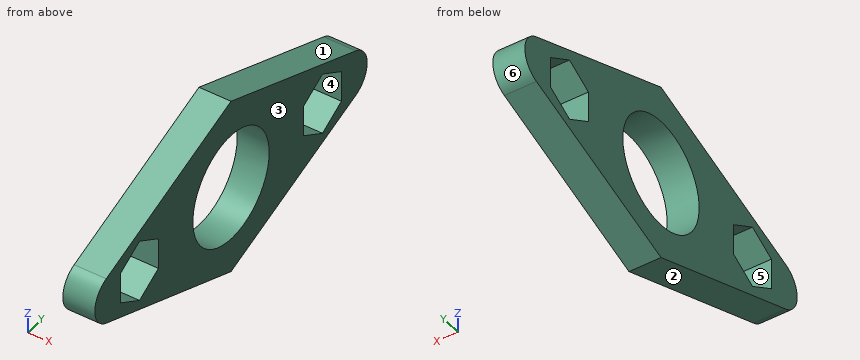
```python
from build123d import *

# Parameters (mm, degrees)
F0_R     = 10.9
F1_DEPTH = 6.35
F2_R     = 5


with BuildPart() as f1:
    # F0 (on Right) → F1 (new body)
    with BuildSketch(Plane.YZ):
        Polygon((48.273511, 0), (0, 18.102249), (-48.273511, 0), (0, -17.76745), align=None)
        Polygon((-20.75447, -3.117691), (-26.15447, -6.235383), (-31.55447, -3.117691), (-31.55447, 3.117691), (-26.15447, 6.235383), (-20.75447, 3.117691), align=None, mode=Mode.SUBTRACT)
        Circle(F0_R, mode=Mode.SUBTRACT)
        Polygon((26.15447, -6.235383), (20.75447, -3.117691), (20.75447, 3.117691), (26.15447, 6.235383), (31.55447, 3.117691), (31.55447, -3.117691), align=None, mode=Mode.SUBTRACT)
    extrude(amount=F1_DEPTH)

    # F2
    f2_edges = [f1.edges().sort_by_distance(p)[0] for p in [
        (3.175, -48.273511, 0),
        (3.175, 48.273511, 0),
    ]]
    fillet(f2_edges, radius=F2_R)


solid = f1.part
```
Can you work these out from the model? Positions are in its coordinate system, mm. Face numbers are marked on the shaded views. A direction names the side the tool comes from. Give positions to 0.01 mm unless a question says otherwise; leave off trailing zeros. Loops run counter-clockwise (first coordinate to the right, second up) from the corner with the lowest first, then second, coordinate; pieces in that order, holes last. Notation, with made-up numbers: M 12,53.25 L 39,53.25 A28 cw 39,77.25 Z; hole C -29,22.25 d9. An arc over 180 degrees is marked long. Use CSV: the item, a comma, the result in double quotes. Start each with the question number.
1. Imagine slicing it at B-B, the plane y = -9.5. Write out the boundary of the cut face in (x, z).
2. If we mould it in two halves opening along Y, with no side actions, what happens to the marked faces 1, 2, 3 and 4? For each: released by +Y, released by -Y, zero draft, split by the parting line, or undercut.
3. If I drill on L1, parallel to Z at x = 5, y = 0; L2, parallel to Z at x = 3.5, y = 31; L3, parallel to Z at x = 5, y = 17, over which ranges is the centre line in solid material (lowest first)?
4. Imagine slicing it at A-A, the plane x = 1. Write out the boundary of the cut face in (y, z), plus the area to 3 significant figures.
5. On a 3-axis mill with a long thin cutter (end or side, diameter ignored), from which of +Z, -Z, +X, -X, +Y, -Y can I reach the whole of each face in a straight line? I mean the marked faces 5 and 6. Say none if no direction works.
6. For P1, Ø1, axis at x = 2.5, y = 15.5, coming from the -Z side; P2, Ø13, axis at y = 0, z = 0, coming from the -X side, each with a flat end and sliding along its axis, tell me the tip position at first contact or that it passes through.
7. Imagine slicing it at D-D, the plane z = 0. Write out the boundary of the cut face in (x, y).
8. Imagine slicing it at C-C, the plane z = 7.5. Write out the boundary of the cut face in (x, y), plus the area to 3 significant figures.
Response values:
1,outline,"M 0,-14.27 L 6.35,-14.27 L 6.35,-5.34 L 0,-5.34 Z; M 0,5.34 L 6.35,5.34 L 6.35,14.54 L 0,14.54 Z"
2,face 1,"released by +Y"
2,face 2,"released by -Y"
2,face 3,"zero draft"
2,face 4,"undercut"
3,L1,"-17.77 to -10.9, 10.9 to 18.1"
3,L2,"-6.36 to -3.44, 3.44 to 6.48"
3,L3,"-11.51 to 11.73"
4,outline,"M -35.67,4.73 A5 ccw -35.64,-4.65 L 0,-17.77 L 35.64,-4.65 A5 ccw 35.67,4.73 L 0,18.1 Z; hole M -31.55,-3.12 L -26.15,-6.24 L -20.75,-3.12 L -20.75,3.12 L -26.15,6.24 L -31.55,3.12 Z; hole C 0,0 d21.8; hole M 20.75,-3.12 L 26.15,-6.24 L 31.55,-3.12 L 31.55,3.12 L 26.15,6.24 L 20.75,3.12 Z"
4,area,"1,080 mm^2"
5,face 5,"+X, -X"
5,face 6,"+X, -X, +Y"
6,P1,"z = -12.25"
6,P2,"through"
7,outline,"M 0,-38.92 L 6.35,-38.92 L 6.35,-31.55 L 0,-31.55 Z; M 0,-20.75 L 6.35,-20.75 L 6.35,-10.9 L 0,-10.9 Z; M 0,10.9 L 6.35,10.9 L 6.35,20.75 L 0,20.75 Z; M 0,31.55 L 6.35,31.55 L 6.35,38.92 L 0,38.92 Z"
8,outline,"M 0,-28.27 L 6.35,-28.27 L 6.35,-7.91 L 0,-7.91 Z; M 0,7.91 L 6.35,7.91 L 6.35,28.27 L 0,28.27 Z"
8,area,"259 mm^2"
